Design review of the part built by this model. Coordinates are the model's own, in mm. Face numbers are marked on the shaded views. Give positions to 0.01 mm unless a question says otherwise; leave off trailing zeros. Write each loop counter-clockwise with the first axis right and the second up, starting at its lowest first coordinate (ties: lowest second). Pieces come first, ordered by that corner, then holes. Notation, with made-up numbers: (45.5, 3.5) -> (58.5, 3.5) arc R27 ccw to (58.5, 22.5) -> close; hole circle Ø10 at (40, 64.5). An arc over 180 degrees is marked (long way). Write each question's results on one line, items separated by ' | '. Start each with the question number.
(1) Take a section at D-D (z = 87). State the section outline as (x, y) points.
(2) To check wall thickness, follow probe 1 along Y at (x, z) = (58.5, 72.5); probe 2 along Z at (x, y) = (-37, -9); probe 3 along Z at (x, y) = (-95, 20). State the ranges of each line that lie inside material, in increasing order.
(3) Mouldability with a two-part tool opening along Z and no side actions: class the marked faces 1, 2 and 3 as released by +Z, released by -Z, zero draft, split by the parting line, or undercut.
(4) Clearance check with flat-ended pins moving along their axes: pin 1 (17.5 mm diameter, centred on y = 2.5, z = 76.5, fed in from +X); pin 2 (19.5 mm diameter, centred on x = 8.12, z = 67.83, fed in from -Y); pin 3 (17.5 mm diameter, centred on y = 6.5, z = 65.5, fed in from -X). State where each tip first meets the part, or that it passes through.
(5) Take a section at C-C (x = -100). State the section outline as (y, z) points.
(6) Take a section at B-B (z = 57). Count the separate pieces of the cut face and the enclosed holes in it, plus the area to 3 significant figures.
(7) Take a section at A-A (y = 28.5). State the section outline as (x, z) points, plus the area to 3 significant figures.
Solid Edge part; units mm, degrees
sketch "Sketch1" plane through (0, 0, 0) normal (0, 0, 1) x (1, 0, 0)
  line L0 (200, -67.5) -> (200, 67.5)
  line L1 (200, 67.5) -> (-200, 67.5)
  line L2 (-200, 67.5) -> (-200, -67.5)
  line L3 (-200, -67.5) -> (200, -67.5)
extrude "Protrusion1" add sketch "Sketch1" along normal blind 22
sketch "Sketch2" plane through (0, 0, 22) normal (0, 0, 1) x (0, 1, 0)
  line L0 (17.5, 75) -> (-17.5, 75)
  line L1 (-17.5, 75) -> (-17.5, 40)
  line L2 (-17.5, 40) -> (17.5, 40)
  line L3 (17.5, 40) -> (17.5, 75)
extrude "Extrusionsausprägung_2" add sketch "Sketch2" along normal blind 20
sketch "Sketch3" plane through (-57.5, -17.5, 32) normal (0, -1, 0) x (1, 0, 0)
  arc A0 (55.7143, 39.8393) -> (59.2857, 39.8393) centre (57.5, 30) cw
  arc A1 (59.2857, 39.8393) -> (70.342, 30) centre (65.6244, 35.8305) cw
  arc A2 (70.342, 30) -> (59.2857, 20.1607) centre (65.6244, 24.1695) cw
  arc A3 (59.2857, 20.1607) -> (55.7143, 20.1607) centre (57.5, 30) cw
  arc A4 (55.7143, 20.1607) -> (44.658, 30) centre (49.3756, 24.1695) cw
  arc A5 (44.658, 30) -> (55.7143, 39.8393) centre (49.3756, 35.8305) cw
  line L0 (17.5, 50) -> (-17.5, 50)
  line L1 (-17.5, 50) -> (-17.5, 10)
  line L2 (-17.5, 10) -> (17.5, 10)
  line L3 (17.5, 10) -> (17.5, 11)
  line L4 (17.5, 11) -> (97.5, 11)
  line L5 (97.5, 11) -> (97.5, 10)
  line L6 (97.5, 10) -> (132.5, 10)
  line L7 (132.5, 10) -> (132.5, 50)
  line L8 (132.5, 50) -> (97.5, 50)
  line L9 (97.5, 50) -> (97.5, 49)
  line L10 (97.5, 49) -> (17.5, 49)
  line L11 (17.5, 49) -> (17.5, 50)
extrude "Extrusionsausprägung_3" add sketch "Sketch3" against normal blind 35
fillet "Verrundung_1" radius 1 4 edges at (-40, 0, 81) (40, 0, 81) (-40, 0, 43) (40, 0, 43)
sketch "Sketch4" plane through (-57.5, 0, 82) normal (0, 0, 1) x (1, 0, 0)
  circle A0 centre (8.5, 0) radius 3
  circle A1 centre (-1, -7) radius 3
  circle A2 centre (-1, 7) radius 3
  circle A3 centre (-10.5, 0) radius 3
  circle A4 centre (106.5, 0) radius 3
  circle A5 centre (116, 7) radius 3
  circle A6 centre (125.5, 0) radius 3
  circle A7 centre (116, -7) radius 3
extrude "Extrusionsausschnitt_1" cut sketch "Sketch4" against normal blind 40
sketch "Sketch5" plane through (57.5, 0, 82) normal (0, 0, 1) x (1, 0, 0)
  line L0 (-17.5, -17.5) -> (-17.5, 17.5)
  line L1 (-17.5, 17.5) -> (17.5, 17.5)
  line L2 (17.5, 17.5) -> (17.5, -17.5)
  line L3 (17.5, -17.5) -> (-17.5, -17.5)
extrude "Extrusionsausprägung_4" add sketch "Sketch5" along normal blind 20
sketch "Sketch6" plane through (57.5, 0, 102) normal (0, 0, 1) x (1, 0, 0)
  line L0 (-257.5, -67.5) -> (142.5, -67.5)
  line L1 (142.5, -67.5) -> (142.5, 67.5)
  line L2 (142.5, 67.5) -> (-257.5, 67.5)
  line L3 (-257.5, 67.5) -> (-257.5, -67.5)
extrude "Extrusionsausprägung_5" add sketch "Sketch6" along normal blind 22
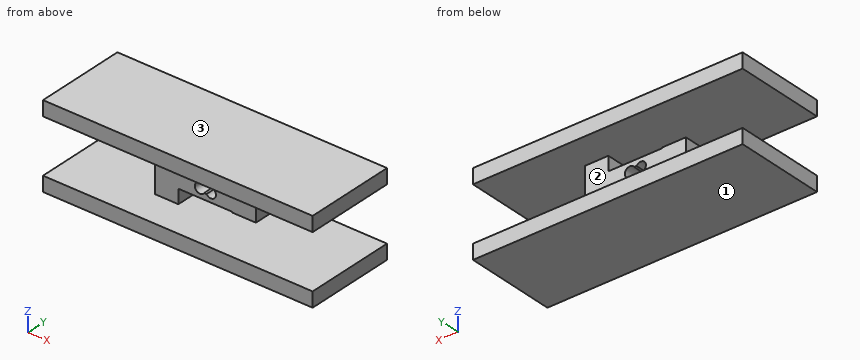
Report:
1) outline: (40, -17.5) -> (75, -17.5) -> (75, 17.5) -> (40, 17.5) -> close
2) probe 1: -17.5 to -10, -4 to 4, 10 to 17.5 | probe 2: 0 to 22, 43 to 81, 102 to 124 | probe 3: 0 to 22, 102 to 124
3) face 1: released by -Z | face 2: undercut | face 3: released by +Z
4) pin 1: x = 75 | pin 2: y = -17.5 | pin 3: x = -75
5) outline: (-67.5, 0) -> (67.5, 0) -> (67.5, 22) -> (-67.5, 22) -> close; (-67.5, 102) -> (67.5, 102) -> (67.5, 124) -> (-67.5, 124) -> close
6) separate pieces: 2 | enclosed holes: 8 | area: 3,930 mm2
7) outline: (-200, 0) -> (200, 0) -> (200, 22) -> (-200, 22) -> close; (-200, 102) -> (200, 102) -> (200, 124) -> (-200, 124) -> close | area: 17,600 mm2
